```python
from build123d import *

# Parameters (mm, degrees)
SKETCH1_W           = 43
SKETCH1_H           = 75
BOSS_EXTRUDE1_DEPTH = 7
CUT_EXTRUDE1_REACH  = 80.334
SKETCH2_R           = 2.5
FILLET1_R           = 0.5
FILLET2_R           = 0.5


with BuildPart() as part:
    # Sketch1 → Boss-Extrude1 (new body)
    with BuildSketch(Plane.XY):
        Rectangle(SKETCH1_W, SKETCH1_H)
    extrude(amount=BOSS_EXTRUDE1_DEPTH)

    # Sketch2 → Cut-Extrude1 (cut, up to next)
    with BuildSketch(Plane(origin=(0, 37.5, 0), x_dir=(1, 0, 0), z_dir=(0, 1, 0)), mode=Mode.PRIVATE) as cut_extrude1_sk1:
        with Locations(Location((0, -3.5, 0), (0, 0, 270))):
            Circle(SKETCH2_R)
    cut_extrude1_tool1 = extrude(cut_extrude1_sk1.sketch, amount=-CUT_EXTRUDE1_REACH, mode=Mode.PRIVATE) & part.part
    add(cut_extrude1_tool1.solids().sort_by_distance((0, 37.5, 3.5))[0], mode=Mode.SUBTRACT)

    # Fillet1
    fillet1_edges = [part.edges().sort_by_distance(p)[0] for p in [
        (-21.5, 0, 7),
        (0, -37.5, 7),
        (21.5, 0, 7),
        (0, -37.5, 0),
        (-21.5, 0, 0),
        (0, 37.5, 0),
        (21.5, 0, 0),
        (0, 37.5, 7),
    ]]
    fillet(fillet1_edges, radius=FILLET1_R)

    # Fillet2
    # the kernel refuses this fillet: 0.5 mm, written as the material it takes off along each edge
    with BuildSketch(Plane(origin=(-21, -37, 6.5), x_dir=(0, -1, 0), z_dir=(-1, 0, 0))) as fillet2_piece_1_section:
        Polygon((0, 0), (FILLET2_R, 0), (FILLET2_R, FILLET2_R), (0, FILLET2_R), align=None)
    fillet2_piece_1 = extrude(amount=FILLET2_R, mode=Mode.PRIVATE)
    fillet2_piece_1 = fillet2_piece_1 - Plane(origin=(-21, -37, 6.5), x_dir=(0, 0.7071067811865475, -0.7071067811865475), z_dir=(-1, 0, 0)) * Sphere(FILLET2_R, mode=Mode.PRIVATE)
    add(fillet2_piece_1, mode=Mode.SUBTRACT)
    with BuildSketch(Plane(origin=(-21, 37, 6.5), x_dir=(-1, 0, 0), z_dir=(0, 1, 0))) as fillet2_piece_2_section:
        Polygon((0, 0), (FILLET2_R, 0), (FILLET2_R, FILLET2_R), (0, FILLET2_R), align=None)
    fillet2_piece_2 = extrude(amount=FILLET2_R, mode=Mode.PRIVATE)
    fillet2_piece_2 = fillet2_piece_2 - Plane(origin=(-21, 37, 6.5), x_dir=(0.7071067811865475, 0, -0.7071067811865475), z_dir=(0, 1, 0)) * Sphere(FILLET2_R, mode=Mode.PRIVATE)
    add(fillet2_piece_2, mode=Mode.SUBTRACT)
    with BuildSketch(Plane(origin=(21, -37, 6.5), x_dir=(0, -1, 0), z_dir=(1, 0, 0))) as fillet2_piece_3_section:
        Polygon((0, 0), (FILLET2_R, 0), (FILLET2_R, -FILLET2_R), (0, -FILLET2_R), align=None)
    fillet2_piece_3 = extrude(amount=FILLET2_R, mode=Mode.PRIVATE)
    fillet2_piece_3 = fillet2_piece_3 - Plane(origin=(21, -37, 6.5), x_dir=(0, 0.7071067811865475, -0.7071067811865475), z_dir=(1, 0, 0)) * Sphere(FILLET2_R, mode=Mode.PRIVATE)
    add(fillet2_piece_3, mode=Mode.SUBTRACT)
    with BuildSketch(Plane(origin=(21, 37, 6.5), x_dir=(1, 0, 0), z_dir=(0, 1, 0))) as fillet2_piece_4_section:
        Polygon((0, 0), (FILLET2_R, 0), (FILLET2_R, -FILLET2_R), (0, -FILLET2_R), align=None)
    fillet2_piece_4 = extrude(amount=FILLET2_R, mode=Mode.PRIVATE)
    fillet2_piece_4 = fillet2_piece_4 - Plane(origin=(21, 37, 6.5), x_dir=(-0.7071067811865475, 0, -0.7071067811865475), z_dir=(0, 1, 0)) * Sphere(FILLET2_R, mode=Mode.PRIVATE)
    add(fillet2_piece_4, mode=Mode.SUBTRACT)
    with BuildSketch(Plane(origin=(21, -37, 0.5), x_dir=(0, -1, 0), z_dir=(1, 0, 0))) as fillet2_piece_5_section:
        Polygon((0, 0), (FILLET2_R, 0), (FILLET2_R, FILLET2_R), (0, FILLET2_R), align=None)
    fillet2_piece_5 = extrude(amount=FILLET2_R, mode=Mode.PRIVATE)
    fillet2_piece_5 = fillet2_piece_5 - Plane(origin=(21, -37, 0.5), x_dir=(0, 0.7071067811865475, 0.7071067811865475), z_dir=(1, 0, 0)) * Sphere(FILLET2_R, mode=Mode.PRIVATE)
    add(fillet2_piece_5, mode=Mode.SUBTRACT)
    with BuildSketch(Plane(origin=(-21, -37, 0.5), x_dir=(0, -1, 0), z_dir=(-1, 0, 0))) as fillet2_piece_6_section:
        Polygon((0, 0), (FILLET2_R, 0), (FILLET2_R, -FILLET2_R), (0, -FILLET2_R), align=None)
    fillet2_piece_6 = extrude(amount=FILLET2_R, mode=Mode.PRIVATE)
    fillet2_piece_6 = fillet2_piece_6 - Plane(origin=(-21, -37, 0.5), x_dir=(0, 0.7071067811865475, 0.7071067811865475), z_dir=(-1, 0, 0)) * Sphere(FILLET2_R, mode=Mode.PRIVATE)
    add(fillet2_piece_6, mode=Mode.SUBTRACT)
    with BuildSketch(Plane(origin=(21, 37, 0.5), x_dir=(1, 0, 0), z_dir=(0, 1, 0))) as fillet2_piece_7_section:
        Polygon((0, 0), (FILLET2_R, 0), (FILLET2_R, FILLET2_R), (0, FILLET2_R), align=None)
    fillet2_piece_7 = extrude(amount=FILLET2_R, mode=Mode.PRIVATE)
    fillet2_piece_7 = fillet2_piece_7 - Plane(origin=(21, 37, 0.5), x_dir=(-0.7071067811865475, 0, 0.7071067811865475), z_dir=(0, 1, 0)) * Sphere(FILLET2_R, mode=Mode.PRIVATE)
    add(fillet2_piece_7, mode=Mode.SUBTRACT)
    with BuildSketch(Plane(origin=(-21, 37, 0.5), x_dir=(-1, 0, 0), z_dir=(0, 1, 0))) as fillet2_piece_8_section:
        Polygon((0, 0), (FILLET2_R, 0), (FILLET2_R, -FILLET2_R), (0, -FILLET2_R), align=None)
    fillet2_piece_8 = extrude(amount=FILLET2_R, mode=Mode.PRIVATE)
    fillet2_piece_8 = fillet2_piece_8 - Plane(origin=(-21, 37, 0.5), x_dir=(0.7071067811865475, 0, 0.7071067811865475), z_dir=(0, 1, 0)) * Sphere(FILLET2_R, mode=Mode.PRIVATE)
    add(fillet2_piece_8, mode=Mode.SUBTRACT)
    with BuildSketch(Plane(origin=(21.5, 37.5, 0.5), x_dir=(-1, 0, 0), z_dir=(0, 0, 1)), Plane(origin=(21.5, -37.5, 0.5), x_dir=(0, 1, 0), z_dir=(0, 0, 1))) as fillet2_piece_9:
        with BuildLine():
            CenterArc((FILLET2_R, FILLET2_R), FILLET2_R, 180, 90)
            Line((0, FILLET2_R), (0, 0))
            Line((0, 0), (FILLET2_R, 0))
        make_face()
    extrude(amount=6, mode=Mode.SUBTRACT)
    with BuildSketch(Plane(origin=(-21.5, -37.5, 0.5), x_dir=(0, 1, 0), z_dir=(0, 0, 1)), Plane(origin=(-21.5, 37.5, 0.5), x_dir=(1, 0, 0), z_dir=(0, 0, 1))) as fillet2_piece_10:
        with BuildLine():
            CenterArc((FILLET2_R, -FILLET2_R), FILLET2_R, 90, 90)
            Line((0, -FILLET2_R), (0, 0))
            Line((0, 0), (FILLET2_R, 0))
        make_face()
    extrude(amount=6, mode=Mode.SUBTRACT)


solid = part.part
```
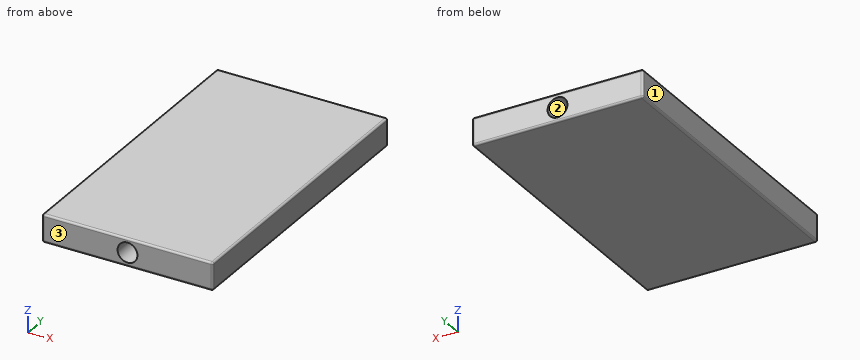
Geometry: final body of the model. Coordinates: model frame, mm. Face numbers are marked on the shaded views. Round coordinates to 2 decimals unless told otherwise and drop trailing zeros. Order: outer loops, then holes, each group sorted by start corner. A loop starts at its lowest first (then second) coordinate and runs counter-clockwise, first axis right, second up. Notation, with made-up numbers: (59.5, -33.75) -> (78.5, -33.75) arc R29 cw to (78.5, -5.75) -> close; hole circle Ø2 at (81.25, 75). An arc over 180 degrees is marked (long way). Use one line per item in the form item = value. Start each with the question number.
1. Draft query along X for the marked faces 1, 2 and 3. Return one class per face: pulls with the +X half, pulls with the -X half, needs draft (parallel to the pull), parting line crosses it, or undercut.
2. Cut plane C-C (y = -19.5). Return the cut outline in (x, z).
3. Line query: probe 1 along X at (y, z) = (5, 3.5); probe 2 along Z at (x, y) = (-1, 32); probe 3 along X at (y, z) = (-24, 2). Output: solid intervals per line, ascending.
4. Cut plane B-B (z = 3.5). Return the cut outline in (x, y), then the cut area to 3 significant figures.
5. Cut plane A-A (x = 0). Return the cut outline in (y, z), then the cut area to 3 significant figures.
Solution:
q1.face_1 = pulls with the -X half
q1.face_2 = undercut
q1.face_3 = needs draft
q2.outline = (-21.5, 0.5) arc R0.5 ccw to (-21, 0) -> (21, 0) arc R0.5 ccw to (21.5, 0.5) -> (21.5, 6.5) arc R0.5 ccw to (21, 7) -> (-21, 7) arc R0.5 ccw to (-21.5, 6.5) -> close; hole circle Ø5 at (0, 3.5)
q3.probe_1 = -21.5 to -2.5, 2.5 to 21.5
q3.probe_2 = 0 to 1.21, 5.79 to 7
q3.probe_3 = -21.5 to -2, 2 to 21.5
q4.outline = (-21.5, -37) arc R0.5 ccw to (-21, -37.5) -> (-2.5, -37.5) -> (-2.5, 37.5) -> (-21, 37.5) arc R0.5 ccw to (-21.5, 37) -> close; (2.5, -37.5) -> (21, -37.5) arc R0.5 ccw to (21.5, -37) -> (21.5, 37) arc R0.5 ccw to (21, 37.5) -> (2.5, 37.5) -> close
q4.area = 2,850 mm^2
q5.outline = (-37.5, 0.5) arc R0.5 ccw to (-37, 0) -> (37, 0) arc R0.5 ccw to (37.5, 0.5) -> (37.5, 1) -> (-37.5, 1) -> close; (-37.5, 6) -> (37.5, 6) -> (37.5, 6.5) arc R0.5 ccw to (37, 7) -> (-37, 7) arc R0.5 ccw to (-37.5, 6.5) -> close
q5.area = 150 mm^2
